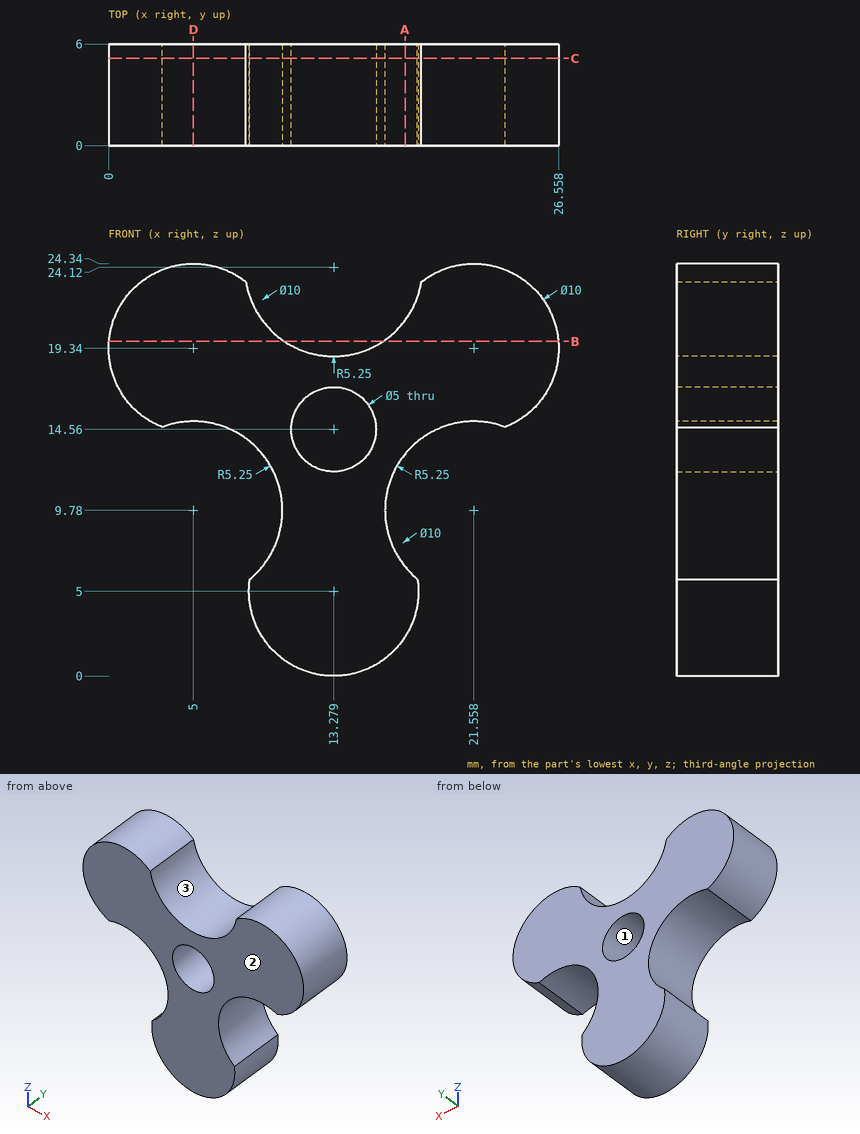
Can you work these out from the drawing? Everything is in mm from the part's minimum corner. Give positions to 0.01 mm unless a question says otherwise; leave off trailing zeros. Order: outer loops, then holes, each group sorted by start corner. A loop starts at its lowest first (then second) coordinate and runs counter-clockwise, first axis right, second up.
Item 1: I need wall thicknesses on line 1 (Z direction, x = 1, y = 0.35); line 2 (Z direction, x = 15.5, y = 0.9) (1 decimal); line 3 (Z direction, x = 10.5, y = 5) (1 decimal). Which ranges of each line are inside material? Lowest first, please.
Item 2: If we section it at D-D, the plane x = 5: Write out the boundary of the cut face in (y, z).
Item 3: If we section it at C-C, the plane y = 5.15: Write out the boundary of the cut face in (x, z), plus the area to 3 significant figures.
Item 4: If we section it at A-A, the plane x = 17.5: Write out the boundary of the cut face in (y, z).
Item 5: I'm going to push flat-ended pins straight in: pin 1 (1.5 mm diameter, centred on x = 18, y = 2, fed in from -Z); pin 2 (2 mm diameter, centred on x = 21.5, z = 19, fed in from -Y); pin 3 (1 mm diameter, centred on y = 3, z = 3, fed in from +X); pin 4 (2 mm diameter, centred on x = 7, y = 1.5, fed in from +Z). Where does each tip first touch, or does it pass through?
Item 6: If we section it at B-B, the plane z = 19.75: Write out the boundary of the cut face in (x, y), plus the area to 3 significant figures.
Item 7: If we mould it in two halves opening along Z, with no side actions, what happens to the marked faces 1, 2 and 3? For each: pulls with the +Z half, pulls with the -Z half, needs draft (parallel to the pull), parting line crosses it, or undercut.
Values:
1. line 1: z = 16.34 to 22.34
1. line 2: z = 0.5 to 13.4, 15.7 to 19.4
1. line 3: z = 0.8 to 19.7
2. outline: (0, 15.03) - (6, 15.03) - (6, 24.34) - (0, 24.34) - close
3. outline: (3.15, 14.69) arc R5.25 cw to (8.33, 5.72) arc R5 ccw (long way) to (18.23, 5.72) arc R5.25 cw to (23.41, 14.69) arc R5 ccw (long way) to (18.46, 23.26) arc R5.25 cw to (8.1, 23.26) arc R5 ccw (long way) to start; hole circle Ø5 at (13.28, 14.56)
3. area: 283 mm2
4. outline: (0, 2.32) - (6, 2.32) - (6, 6.45) - (0, 6.45) - close; (0, 13.11) - (6, 13.11) - (6, 21) - (0, 21) - close
5. pin 1: stops at z = 1.96
5. pin 2: stops at y = 0
5. pin 3: stops at x = 18.05
5. pin 4: stops at z = 24.24
6. outline: (0.02, 0) - (10.37, 0) - (10.37, 6) - (0.02, 6) - close; (16.19, 0) - (26.54, 0) - (26.54, 6) - (16.19, 6) - close
6. area: 124 mm2
7. face 1: undercut
7. face 2: needs draft
7. face 3: pulls with the +Z half
